Part model, mm, in its own coordinate system. A direction names the side the tool comes from. Coordinates: 2 decimals unless noted, no trailing zeros. Write each loop counter-clockwise with the first axis right and the second up, starting at its lowest first coordinate (ties: lowest second). Pieces come first, ordered by that corner, then holes. Notation, with made-up numbers: (-4, 34) -> (3, 34) arc R31 ccw to (3, 59) -> close; hole circle Ø1 at (-4, 86.25). An arc over 180 degrees is marked (long way). One line per question, with ' | ' between items. Start each with the question number.
Item 1: Pin check, flat tips, straight feed: pin 1 (14.5 mm diameter, centred on y = -72, z = 96, fed in from -X); pin 2 (14.5 mm diameter, centred on x = -1, z = 102, fed in from -Y); pin 3 (2 mm diameter, centred on x = -4.5, y = -33, fed in from +Z). Stop position of each tip, or through.
Item 2: Saw through at A-A (x = 0). List the corners of the cut face in (y, z).
Item 3: Probe probe 1 along Z at (x, y) = (-38.5, -48.5); probe 2 along Y at (x, z) = (-26.5, -112); probe 3 along X at (y, z) = (-69.5, -77.5). List the from-to ranges inside material, lowest first. Write a range as [from, to].
Item 4: 3-axis set-ups, long thin cutter, end or side, ignore diameter. For faces 5 (the cylindrical face through (1.573, -118.58, -101.094)), 6 (the flat face through (88, 10, 88)), 7 (the flat face through (-1, -29, -32.035)): which of +Z, -Z, +X, -X, +Y, -Y reach the whole face in a straight line?
Item 5: Saw through at D-D (y = -51). List the corners of the cut face in (x, z), and give its area (3 significant figures).
Item 6: Saw through at C-C (z = 103). List the corners of the cut face in (x, y), and give its area (3 significant figures).
Item 7: Saw through at B-B (y = 42). List the corners of the cut face in (x, z), and give its area (3 significant figures).
Item 8: Two-plate mould, pull along X, no slides. Class faces 1 (the flat face through (-21, -112.496, 49)), 2 (the flat face through (1, -124.496, -24)), 3 (the flat face through (-88, -26, 22)), 4 (the flat face through (100, -26, 2)): pulls with the +X half, pulls with the -X half, needs draft (parallel to the pull), parting line crosses it, or undercut.
from build123d import *

# Parameters (mm, degrees)
F1_DEPTH = 100
F2_T     = -12
F3_W     = 176
F3_H     = 12
F4_DEPTH = 188
F6_DEPTH = 12


with BuildPart() as f1:
    # F0 (on Right) → F1 (new body, symmetric)
    with BuildSketch(Plane.YZ):
        Polygon((-124.4957186917, 75.0704253932), (-124.4957186917, -124.9295746068), (75.5042813083, -124.9295746068), (75.5042813083, 125.0704253932), align=None)
    extrude(amount=F1_DEPTH, both=True)

    # F2
    f2_openings = [f1.faces().sort_by_distance(p)[0] for p in [
        (0, -124.495719, -24.929575),
        (0, -24.495719, 100.070425),
    ]]
    offset(amount=F2_T, openings=f2_openings)

    # F3 (on face) → F4 (join)
    with BuildSketch(Plane.XZ.offset(-63.5042813083)):
        with Locations((0, -26.0345488787)):
            Rectangle(F3_W, F3_H)
        with Locations((0, 68.4323040247)):
            Rectangle(F3_W, F3_H)
    extrude(amount=F4_DEPTH)

    # F5 (on face) → F6 (join)
    with BuildSketch(Plane.XZ.offset(124.4957186917)):
        Polygon((100, -124.9295746068), (100, 75.0704253932), (88, 75.0704253932), (88, 74.4323040247), (-88, 74.4323040247), (-88, 75.0704253932), (-100, 75.0704253932), (-100, -124.9295746068), align=None)
        Polygon((88, -112.9295746068), (-88, -112.9295746068), (-88, -32.0345488787), (-88, -20.0345488787), (-88, 62.4323040247), (88, 62.4323040247), (88, -20.0345488787), (88, -32.0345488787), align=None, mode=Mode.SUBTRACT)
        with BuildLine():
            Line((-88, 62.4323040247), (-88, -20.0345488787))
            Line((-88, -20.0345488787), (-75.6174618507, -20.0345488787))
            ThreePointArc((-75.6174618507, -20.0345488787), (0, 50.4918066225), (75.6174618507, -20.0345488787))
            Line((75.6174618507, -20.0345488787), (88, -20.0345488787))
            Line((88, -20.0345488787), (88, 62.4323040247))
            Line((88, 62.4323040247), (-88, 62.4323040247))
        make_face()
        with BuildLine():
            Line((-88, -32.0345488787), (-88, -112.9295746068))
            Line((-88, -112.9295746068), (88, -112.9295746068))
            Line((88, -112.9295746068), (88, -32.0345488787))
            Line((88, -32.0345488787), (75.5022996144, -32.0345488787))
            ThreePointArc((75.5022996144, -32.0345488787), (0, -101.1106302402), (-75.5022996144, -32.0345488787))
            Line((-75.5022996144, -32.0345488787), (-88, -32.0345488787))
        make_face()
    extrude(amount=-F6_DEPTH)


solid = f1.part
From the geometry:
1) pin 1: through | pin 2: y = 63.5 | pin 3: z = 74.43
2) outline: (-124.5, -124.93) -> (75.5, -124.93) -> (75.5, 125.07) -> (63.5, 122.07) -> (63.5, 74.43) -> (-124.5, 74.43) -> (-124.5, 50.49) -> (-112.5, 50.49) -> (-112.5, 62.43) -> (63.5, 62.43) -> (63.5, -20.03) -> (-124.5, -20.03) -> (-124.5, -32.03) -> (63.5, -32.03) -> (63.5, -112.93) -> (-112.5, -112.93) -> (-112.5, -101.11) -> (-124.5, -101.11) -> close
3) probe 1: [-124.93, -112.93], [-32.03, -20.03], [62.43, 74.43] | probe 2: [-124.5, -112.5], [63.5, 75.5] | probe 3: [-100, -88], [88, 100]
4) face 5: -Y | face 6: +Z, -Y | face 7: none
5) outline: (-100, -124.93) -> (100, -124.93) -> (100, 93.44) -> (88, 93.44) -> (88, 74.43) -> (-88, 74.43) -> (-88, 93.44) -> (-100, 93.44) -> close; hole (-88, -112.93) -> (88, -112.93) -> (88, -32.03) -> (-88, -32.03) -> close; hole (-88, -20.03) -> (88, -20.03) -> (88, 62.43) -> (-88, 62.43) -> close | area: 11,600 mm2
6) outline: (-100, -12.78) -> (-88, -12.78) -> (-88, 63.5) -> (88, 63.5) -> (88, -12.78) -> (100, -12.78) -> (100, 75.5) -> (-100, 75.5) -> close | area: 4,230 mm2
7) outline: (-100, -124.93) -> (100, -124.93) -> (100, 116.69) -> (88, 116.69) -> (88, 74.43) -> (-88, 74.43) -> (-88, 116.69) -> (-100, 116.69) -> close; hole (-88, -112.93) -> (88, -112.93) -> (88, -32.03) -> (-88, -32.03) -> close; hole (-88, -20.03) -> (88, -20.03) -> (88, 62.43) -> (-88, 62.43) -> close | area: 12,100 mm2
8) face 1: undercut | face 2: needs draft | face 3: undercut | face 4: pulls with the +X half
